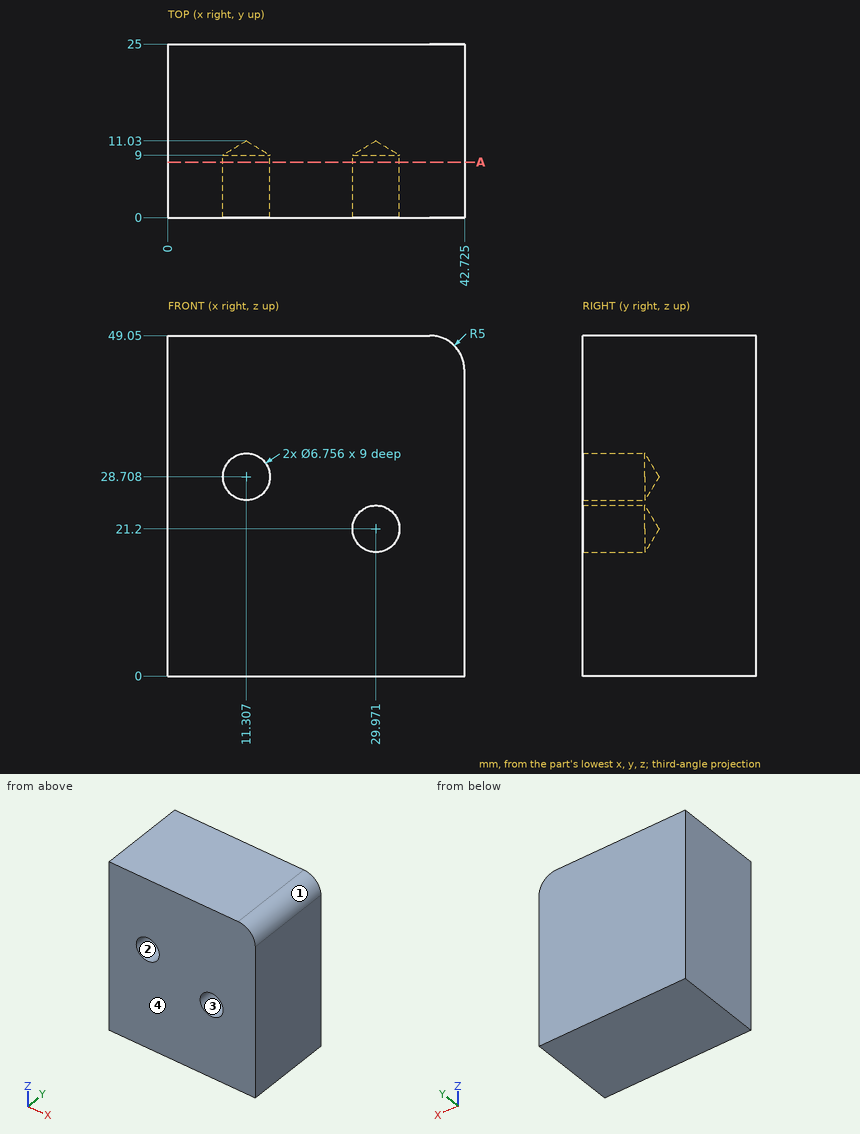
Input: dimensioned drawing with shaded views. Units: mm. Origin: part minimum x, y, z. Coordinates: 2 decimals unless noted, no trailing zeros. Use a Markdown table: item, result. Add a question column.
Q1. Section query A-A, the plane y = 8. State how many separate pieces and enclosed holes the cut face has, and give its area (3 significant figures).
Q2. Material intervals for L1, parallel to Z at x = 38, y = 13.25; L2, parallel to X at y = 8, z = 19 (1 decimal); L3, parallel to X at y = 2.75, z = 28 (1 decimal), sorted ascending.
Q3. First-contact query: pin 1 (3 mm diameter, centred on x = 29, z = 8, fed in from -Y); pin 2 (4 mm diameter, centred on x = 29.97, z = 21.2, fed in from -Y). Flat tips, straight axial feed; report the tip coordinate or a pass-through.
Q4. Draft query along X for the marked faces 1, 2, 3 and 4. Return one class per face: pulls with the +X half, pulls with the -X half, needs draft (parallel to the pull), parting line crosses it, or undercut.
Result:
| question | item | result |
|---|---|---|
| 1 | separate pieces | 1 |
| 1 | enclosed holes | 2 |
| 1 | area | 2,020 mm2 |
| 2 | L1 | z = 0 to 49.04 |
| 2 | L2 | x = 0 to 27.4, 32.5 to 42.7 |
| 2 | L3 | x = 0 to 8, 14.6 to 42.7 |
| 3 | pin 1 | stops at y = 0 |
| 3 | pin 2 | stops at y = 9.83 |
| 4 | face 1 | pulls with the +X half |
| 4 | face 2 | undercut |
| 4 | face 3 | undercut |
| 4 | face 4 | needs draft |
